The listing builds one solid part. Answer for the finished solid, in the listing's coordinates (mm). A direction names the side the tool comes from. Round coordinates to 2 decimals unless told otherwise and drop trailing zeros. Loops run counter-clockwise (first coordinate to the right, second up) from the corner with the lowest first, then second, coordinate; pieces in that order, holes last. Notation, with made-up numbers: (56, -4.75) -> (87, -4.75) arc R3 ccw to (87, -0.75) -> close; hole circle Ø10 at (88, 41.25). An arc over 180 degrees is marked (long way). One line per question, with ' | ' between items.
from build123d import *

# Parameters (mm, degrees)
SKETCH1_W           = 38.1
SKETCH1_H           = 24.003
BOSS_EXTRUDE1_DEPTH = 12.7
SKETCH3_R           = 4.445
FILLET1_R           = 3.81


with BuildPart() as part:
    # Sketch1 → Boss-Extrude1 (new body)
    with BuildSketch(Plane(origin=(0, 0, 0), x_dir=(0, 1, 0), z_dir=(0, 0, 1))):
        Rectangle(SKETCH1_W, SKETCH1_H)
    extrude(amount=BOSS_EXTRUDE1_DEPTH)

    # Sweep1: sweep along a path in Sketch2
    with BuildLine(Plane(origin=(5.6515, 0, 0), x_dir=(0, 0, -1), z_dir=(1, 0, 0))) as sweep1_path:
        Line((-6.35, 19.05), (-6.35, 38.735))
        ThreePointArc((-6.35, 38.735), (-9.139807909, 45.470192091), (-15.875, 48.26))
        Line((-15.875, 48.26), (-88.9, 48.26))
    # Sketch3 → Sweep1 (sweep)
    with BuildSketch(Plane(origin=(0, 19.05, 0), x_dir=(-1, 0, 0), z_dir=(0, 1, 0))):
        with Locations((-5.6515, 6.35)):
            Circle(SKETCH3_R)
    sweep(path=sweep1_path.line)

    # Fillet1
    fillet1_edges = [part.edges().sort_by_distance(p)[0] for p in [
        (10.0965, 48.26, 88.9),
    ]]
    fillet(fillet1_edges, radius=FILLET1_R)


solid = part.part
Q1. A cutting plane is placed at C-C on z = 66.5. Give the vertices of the cut face in (x, y) (1 decimal).
Numbers:
outline: circle Ø8.9 at (5.7, 48.3)
Q2. For faces 1 (the face through (0, 0, 12.7)), 2 (the face through (12.002, 0, 6)), determine the directions among +Z, -Z, +X, -X, +Y, -Y from which every point of the face is accessible in a straight line to the end or side of a thin tool.
Numbers:
face 1: +Z, +X, -X, -Y | face 2: +Z, -Z, +X, +Y, -Y
Q3. Given pin 1 Ø10 at (x, z) = (5, 4.5) entering from +Y; pin 2 Ø10 at (x, y) = (4.5, 32.5) entering from -Z (3 decimals); pin 3 Ø12 at (x, z) = (8.5, 10.5) entering from +Y, each flat-ended and moving along its own axis, determine where each tip first touches the part or whether it passes through.
Numbers:
pin 1: y = 51.15 | pin 2: z = 1.905 | pin 3: y = 52.7
Q4. Find the intervals of material crossed by line 1 (Z direction, x = -8, y = -10.5); line 2 (Y direction, x = 6, z = 73.5); line 3 (Y direction, x = 3.25, z = 52), in increasing order. Write a range as from..to.
Numbers:
line 1: 0..12.7 | line 2: 43.83..52.69 | line 3: 44.52..52
Q5. For a pull along Y with two mould halves and no side action, classify faces 3 (the face through (0, -19.05, 6)), 4 (the face through (1.412, 29.03, 7.685)), 5 (the face through (-12.002, 0, 6)), 6 (the face through (1.412, 46.925, 50.967)) as pulls with the +Y half, pulls with the -Y half, needs draft (parallel to the pull), parting line crosses it, or undercut.
Numbers:
face 3: pulls with the -Y half | face 4: undercut | face 5: needs draft | face 6: parting line crosses it
Q6. A cutting plane is placed at A-A on x = -7. Give the vertices of the cut face in (y, z).
Numbers:
outline: (-19.05, 0) -> (19.05, 0) -> (19.05, 12.7) -> (-19.05, 12.7) -> close
Q7. A cutting plane is placed at B-B on y = -3. Give the vertices of the cut face in (x, z).
Numbers:
outline: (-12, 0) -> (12, 0) -> (12, 12.7) -> (-12, 12.7) -> close
